```python
from build123d import *

# Parameters (mm, degrees)
Y_KSEKLIK_EKSTR_ZYON1_DEPTH = 20
IZIM2_R                     = 6
KES_EKSTR_ZYON1_DEPTH       = 92.651513899


with BuildPart() as part:
    # Çizim1 → Yükseklik-Ekstrüzyon1 (new body)
    with BuildSketch(Plane.XY):
        with BuildLine():
            Line((-30, -24), (-30, 0))
            Line((-30, 0), (-24, 0))
            ThreePointArc((-24, 0), (0, 24), (24, 0))
            Line((24, 0), (30, 0))
            Line((30, 0), (30, -24))
            Line((30, -24), (24, -24))
            Line((24, -24), (24, -36))
            Line((24, -36), (33, -36))
            Line((33, -36), (40, -36))
            Line((40, -36), (40, -11.038880633))
            Line((40, -11.038880633), (40, 0))
            Line((40, 0), (36, 0))
            ThreePointArc((36, 0), (28.525322537, 21.961465665), (9.205223658, 34.803216193))
            Line((9.205223658, 34.803216193), (9.205223658, 44))
            Line((9.205223658, 44), (-9.33749561, 44))
            Line((-9.33749561, 44), (-9.33749561, 34.767961915))
            ThreePointArc((-9.33749561, 34.767961915), (-28.567025064, 21.907192404), (-36, 0))
            Line((-36, 0), (-40, 0))
            Line((-40, 0), (-40, -11.038880633))
            Line((-40, -11.038880633), (-40, -36))
            Line((-40, -36), (-33.54247299, -36))
            Line((-33.54247299, -36), (-24, -36))
            Line((-24, -36), (-24, -24))
            Line((-24, -24), (-30, -24))
        make_face()
    extrude(amount=Y_KSEKLIK_EKSTR_ZYON1_DEPTH)

    # Çizim2 → Kes-Ekstrüzyon1 (cut, through all)
    with BuildSketch(Plane(origin=(0, 44, 0), x_dir=(1, 0, 0), z_dir=(0, 1, 0))):
        with Locations(Location((0, -10, 0), (0, 0, 270))):
            Circle(IZIM2_R)
    extrude(amount=-KES_EKSTR_ZYON1_DEPTH, mode=Mode.SUBTRACT)


solid = part.part
```
Work out the finished part from the listing and answer in its coordinate system (mm). A direction names the side the tool comes from. Coordinates: 2 decimals unless noted, no trailing zeros. Write each loop counter-clockwise with the first axis right and the second up, starting at its lowest first coordinate (ties: lowest second). Pieces come first, ordered by that corner, then holes.
Q1. A cutting plane is placed at A-A, the plane y = -25.5. Give the vertices of the cut face in (x, z).
Q2. Which of the six approach directions +Z, -Z, +X, -X, +Y, -Y give full straight-line access (tool end or side, diameter ignored) to faces 1 (the face through (-27, 0, 10)), 2 (the face through (38, 0, 10)), 3 (the face through (-9.337, 39, 10)), 4 (the face through (-24, -30, 10))?
Q3. A cutting plane is placed at D-D, the plane z = 3. Give the vertices of the cut face in (x, y), then the cut area to 3 significant figures.
Q4. A cutting plane is placed at C-C, the plane z = 10. Give the vertices of the cut face in (x, y), then the cut area to 3 significant figures.
Q5. Find the intervals of material crossed by line 1 (X direction, y = -21, z = 15.25); line 2 (Z direction, x = 0, y = 36.75); line 3 (X direction, y = 39.75, z = 10), in increasing order.
Q6. Each of these flat-tipped pins is pushed along its axis until it touches: pin 1 Ø4 at (x, z) = (-6, 6.5) entering from -Y; pin 2 Ø2 at (y, z) = (1.5, 6.5) entering from -X; pin 3 Ø5 at (x, z) = (27.5, 7) entering from +Y. Where does it stop, or does it pass through?
Q7. A cutting plane is placed at B-B, the plane x = 0. Give the vertices of the cut face in (y, z), then the cut area to 3 significant figures.
Q8. Determine the mould class of faces 5 (the face through (27, -24, 10)), 6 (the face through (30, -12, 10)), 7 (the face through (-8.702, 22.367, 9.86)), 8 (the face through (-28.365, 22.168, 9.86)) for opening direction Y: released by +Y, released by -Y, zero draft, split by the parting line, or undercut.
Findings below:
1. outline: (-40, 0) - (-24, 0) - (-24, 20) - (-40, 20) - close; (24, 0) - (40, 0) - (40, 20) - (24, 20) - close
2. face 1: +Z, -Z
2. face 2: +Z, -Z, +X, +Y
2. face 3: +Z, -Z, -X, +Y
2. face 4: +Z, -Z, -Y
3. outline: (-40, -36) - (-24, -36) - (-24, -24) - (-30, -24) - (-30, 0) - (-24, 0) arc R24 cw to (24, 0) - (30, 0) - (30, -24) - (24, -24) - (24, -36) - (40, -36) - (40, 0) - (36, 0) arc R36 ccw to (9.21, 34.8) - (9.21, 44) - (-9.34, 44) - (-9.34, 34.77) arc R36 ccw to (-36, 0) - (-40, 0) - close
3. area: 2,150 mm2
4. outline: (-40, -36) - (-24, -36) - (-24, -24) - (-30, -24) - (-30, 0) - (-24, 0) arc R24 cw to (-6, 23.24) - (-6, 44) - (-9.34, 44) - (-9.34, 34.77) arc R36 ccw to (-36, 0) - (-40, 0) - close; (6, 23.24) arc R24 cw to (24, 0) - (30, 0) - (30, -24) - (24, -24) - (24, -36) - (40, -36) - (40, 0) - (36, 0) arc R36 ccw to (9.21, 34.8) - (9.21, 44) - (6, 44) - close
4. area: 1,910 mm2
5. line 1: x = -40 to -30, 30 to 40
5. line 2: z = 0 to 4, 16 to 20
5. line 3: x = -9.34 to -6, 6 to 9.21
6. pin 1: stops at y = 22.63
6. pin 2: stops at x = -36
6. pin 3: stops at y = 25.9
7. outline: (24, 0) - (44, 0) - (44, 4) - (24, 4) - close; (24, 16) - (44, 16) - (44, 20) - (24, 20) - close
7. area: 160 mm2
8. face 5: undercut
8. face 6: undercut
8. face 7: released by -Y
8. face 8: released by +Y
